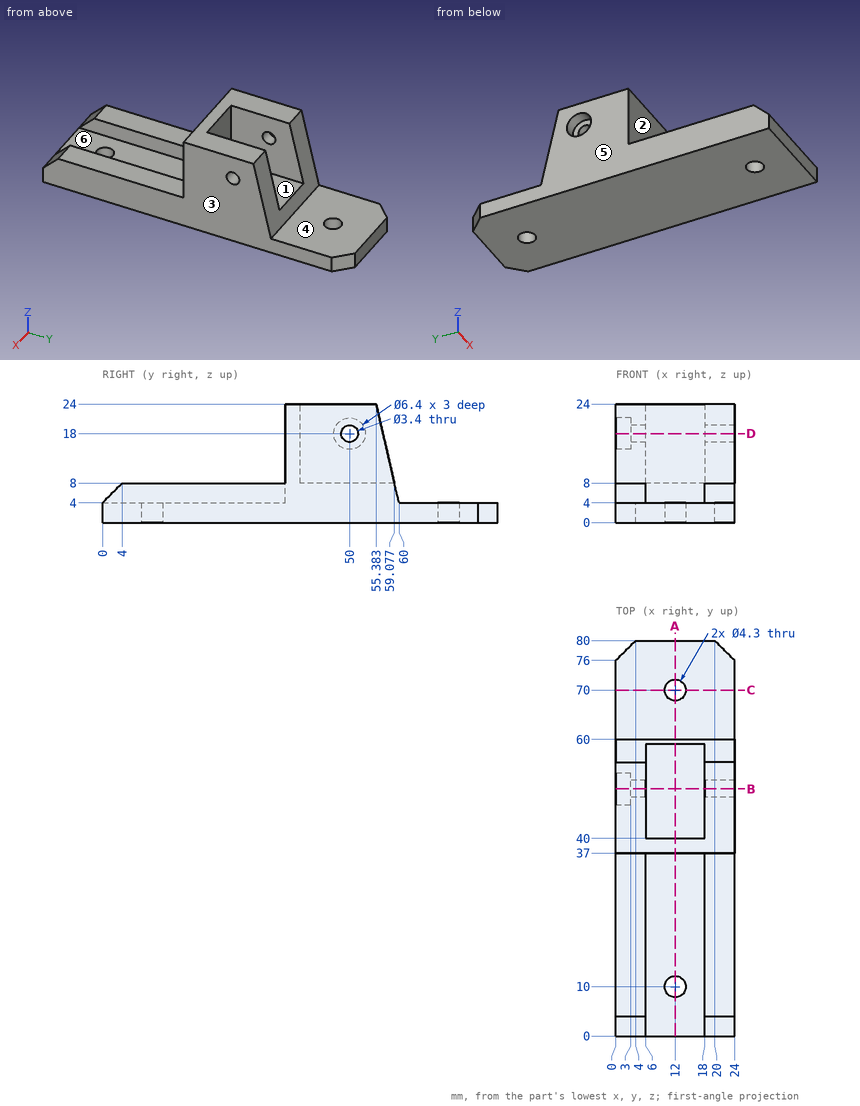
Job drawing, mm, ordinate dimensions from the low corner. One solid piece. A direction names the side the tool comes from. Coordinates: 2 decimals unless noted, no trailing zeros. Write each loop counter-clockwise with the first axis right and the second up, starting at its lowest first coordinate (ties: lowest second). Pieces come first, ordered by that corner, then holes. Notation, with made-up numbers: M 24.25,10.25 L 77.25,10.25 A33 ccw 77.25,49.25 Z; hole C -12,-39.5 d4. An arc over 180 degrees is marked long. Answer as a JSON object with one key per item and string values. Group by question number.
1) Pin check, flat tips, straight feed: pin 1 Ø3 at (x, z) = (16.5, 20.5) entering from -Y; pin 2 Ø6 at (x, z) = (20, 10) entering from +Y; pin 3 Ø1.8 at (x, y) = (2.5, 22) entering from +Z. Stop position of each tip, or through.
2) Saw through at A-A (x = 12). Give the number of separate pieces and of enclosed holes in the cut face, plus the area to 3 significant figures.
3) Saw through at D-D (z = 18). Write the cut outline in (x, y).
4) Saw through at C-C (y = 70). Write the cut outline in (x, z), plus the area to 3 significant figures.
5) Tool access for the marked faces 1, 2 and 3: list every direction of +Z, -Z, +X, -X, +Y, -Y with a clear straight run to the whole face (end or side of a thin tool).
6) Mould opens along X. For the marked faces 4, 5 and 6 say: +X half, -X half, draft (parallel to the pull), parting line (faces both ways), or undercut.
7) Saw through at B-B (y = 50). Write the cut outline in (x, z).
8) Wall check: line 1 (Y direction, x = 12, z = 1.7); line 2 (X direction, y = 44, z = 14.5); line 3 (Z direction, x = 0.95, y = 50). Give the ranges that are in metal, low to high. Write a range as from..to.
Values follow:
{
 "1": {"pin 1": "stops at y = 37", "pin 2": "stops at y = 59.31", "pin 3": "stops at z = 8"},
 "2": {"separate pieces": "3", "enclosed holes": "0", "area": "424 mm2"},
 "3": {"outline": "M 0,37 L 24,37 L 24,48.3 L 18,48.3 L 18,40 L 6,40 L 6,48.3 L 3,48.3 L 3,46.8 L 0,46.8 Z; M 0,53.2 L 3,53.2 L 3,51.7 L 6,51.7 L 6,56.77 L 0,56.77 Z; M 18,51.7 L 24,51.7 L 24,56.77 L 18,56.77 Z"},
 "4": {"outline": "M 0,0 L 9.85,0 L 9.85,4 L 0,4 Z; M 14.15,0 L 24,0 L 24,4 L 14.15,4 Z", "area": "78.8 mm2"},
 "5": {"face 1": "+Z, +Y", "face 2": "+Z, -Y", "face 3": "+Z, -Z, +X, +Y, -Y"},
 "6": {"face 4": "draft", "face 5": "-X half", "face 6": "undercut"},
 "7": {"outline": "M 0,0 L 24,0 L 24,16.3 L 18,16.3 L 18,8 L 6,8 L 6,16.3 L 3,16.3 L 3,14.8 L 0,14.8 Z; M 0,21.2 L 3,21.2 L 3,19.7 L 6,19.7 L 6,24 L 0,24 Z; M 18,19.7 L 24,19.7 L 24,24 L 18,24 Z"},
 "8": {"line 1": "y = 0..7.85, 12.15..67.85, 72.15..80", "line 2": "x = 0..6, 18..24", "line 3": "z = 0..14.8, 21.2..24"}
}
